Build history of the part. All positions in model axes, mm. Round coordinates to 2 decimals unless told otherwise and drop trailing zeros. Order: outer loops, then holes, each group sorted by start corner. A loop starts at its lowest first (then second) coordinate and runs counter-clockwise, first axis right, second up. Notation, with made-up numbers: (37, 59.25) -> (80, 59.25) arc R15 cw to (80, 67.25) -> close; hole circle Ø4 at (59.5, 73). An arc over 180 degrees is marked (long way). Answer as CSV lines item,"result". Start each with the question number.
```python
from build123d import *

# Parameters (mm, degrees)
BOSS_EXTRUDE1_DEPTH = 2.7
FILLET6_R           = 1
FILLET7_R           = 2


with BuildPart() as part:
    # Sketch1 → Boss-Extrude1 (new body)
    with BuildSketch(Plane(origin=(0, 0, 0), x_dir=(1, 0, 0), z_dir=(0, 1, 0))):
        Polygon((-14.25, 15.125), (-18.5, 15.125), (-18.5, 22.375), (18.5, 22.375), (18.5, 15.125), (14.25, 15.125), (14.25, -15.125), (-14.25, -15.125), align=None)
    extrude(amount=BOSS_EXTRUDE1_DEPTH)

    # Fillet6
    fillet6_edges = [part.edges().sort_by_distance(p)[0] for p in [
        (14.25, 1.35, 15.125),
        (-14.25, 1.35, 15.125),
        (-18.5, 1.35, -15.125),
        (-18.5, 1.35, -22.375),
        (18.5, 1.35, -22.375),
        (18.5, 1.35, -15.125),
    ]]
    fillet(fillet6_edges, radius=FILLET6_R)

    # Fillet7
    fillet7_edges = [part.edges().sort_by_distance(p)[0] for p in [
        (14.25, 1.35, -15.125),
        (-14.25, 1.35, -15.125),
    ]]
    fillet(fillet7_edges, radius=FILLET7_R)


solid = part.part
```
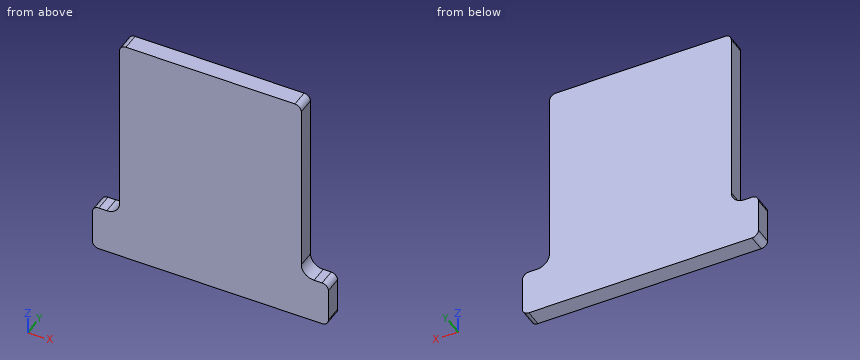
Q1. Slice it at A-A, the plane y = 1.7. Write the cut outline in (x, z) (3 decimals).
Q2. Probe L1, parallel to X at y = 1.3, z = -12; L2, parallel to X at y = 0.8, z = -16; L3, parallel to Z at x = 15, y = 0.65 (3 decimals). List the from-to ranges inside material, lowest first.
Q3. Flat gauge pins, fed straight in: pin 1 Ø0.6 at (x, y) = (16.5, 0.5) entering from +Z; pin 2 Ø1.4 at (y, z) = (2, 1) entering from +X. Where does each tip first touch, or does it go through?
Q4. Slice it at B-B, the plane z = 10. Write the cut outline in (x, y), plus the area to 4 significant figures.
Q5. Slice it at C-C, the plane x = 15.5. Write the cut outline in (y, z) (3 decimals), plus the area to 3 significant figures.
Solutions:
1,outline,"(-18.5, -21.375) arc R1 ccw to (-17.5, -22.375) -> (17.5, -22.375) arc R1 ccw to (18.5, -21.375) -> (18.5, -16.125) arc R1 ccw to (17.5, -15.125) -> (16.25, -15.125) arc R2 cw to (14.25, -13.125) -> (14.25, 14.125) arc R1 ccw to (13.25, 15.125) -> (-13.25, 15.125) arc R1 ccw to (-14.25, 14.125) -> (-14.25, -13.125) arc R2 cw to (-16.25, -15.125) -> (-17.5, -15.125) arc R1 ccw to (-18.5, -16.125) -> close"
2,L1,"x = -14.25 to 14.25"
2,L2,"x = -18.49 to 18.49"
2,L3,"z = -22.375 to -14.686"
3,pin 1,"stops at z = -15.12"
3,pin 2,"stops at x = 14.25"
4,outline,"(-14.25, 0) -> (14.25, 0) -> (14.25, 2.7) -> (-14.25, 2.7) -> close"
4,area,"76.95 mm2"
5,outline,"(0, -22.375) -> (2.7, -22.375) -> (2.7, -14.979) -> (0, -14.979) -> close"
5,area,"20.0 mm2"
